Input: part model. Units: mm. Frame: model coordinates. Face numbers are marked on the shaded views. A direction names the side the tool comes from. Coordinates: 2 decimals unless noted, no trailing zeros. Order: outer loops, then holes, each group sorted by start corner. A loop starts at its lowest first (then second) coordinate and runs counter-clockwise, first axis right, second up. Notation, with made-up numbers: M -24.5,-1 L -4.5,-1 A7 cw -4.5,6 Z; hole C -3.5,28 d5. An arc over 180 degrees is marked long. Answer in a Markdown table with one row per item.
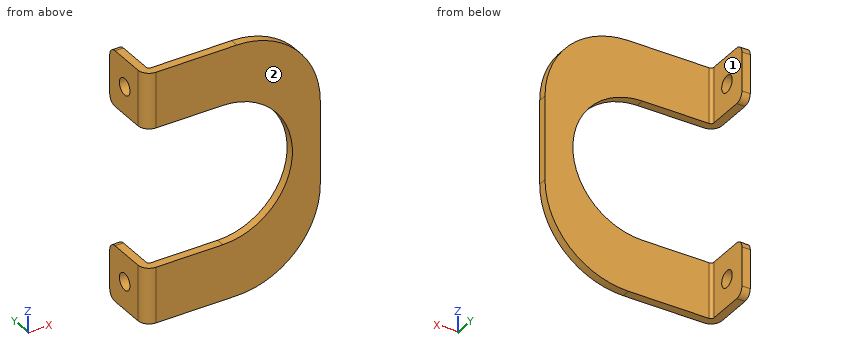
from build123d import *

# Parameters (mm, degrees)
BOSS_EXTRUDE1_DEPTH            = 3
EDGE_FLANGE1_STRIP_W           = 14
EDGE_FLANGE1_STRIP_H           = 3
EDGE_FLANGE1_STRIP_CUT_DEPTH   = 20
EDGE_FLANGE1_STRIP_2_W         = 14
EDGE_FLANGE1_STRIP_2_H         = 3
EDGE_FLANGE1_STRIP_CUT_2_DEPTH = 20
EDGE_FLANGE1_DEPTH             = 20
EDGE_FLANGE1_BEND_DEPTH        = 20
FILLET1_R                      = 3
CUT_EXTRUDE1_REACH             = 79.621
SKETCH12_R                     = 3


# Sheet-metal steps are written as plain solids
with BuildPart() as part:
    # Sketch1 → Boss-Extrude1 (new body)
    with BuildSketch(Plane(origin=(0, 0, 0), x_dir=(1, 0, 0), z_dir=(0, 1, 0))):
        with BuildLine():
            Line((0, 25), (-25, 25))
            Line((-25, 25), (-25, 45))
            Line((-25, 45), (5, 45))
            ThreePointArc((5, 45), (26.213203436, 36.213203436), (35, 15))
            Line((35, 15), (35, -15))
            ThreePointArc((35, -15), (26.213203436, -36.213203436), (5, -45))
            Line((5, -45), (-25, -45))
            Line((-25, -45), (-25, -25))
            Line((-25, -25), (0, -25))
            ThreePointArc((0, -25), (25, 0), (0, 25))
        make_face()
    extrude(amount=BOSS_EXTRUDE1_DEPTH)

    # Edge-Flange1 strip (across the edge) → Edge-Flange1 strip cut (cut)
    with BuildSketch(Plane(origin=(-25, 3, 25), x_dir=(1, 0, 0), z_dir=(0, 0, 1))):
        with Locations((-6, -1.5)):
            Rectangle(EDGE_FLANGE1_STRIP_W, EDGE_FLANGE1_STRIP_H)
    extrude(amount=EDGE_FLANGE1_STRIP_CUT_DEPTH, mode=Mode.SUBTRACT)

    # Edge-Flange1 strip 2 (across the edge) → Edge-Flange1 strip cut 2 (cut)
    with BuildSketch(Plane(origin=(-25, 3, -45), x_dir=(1, 0, 0), z_dir=(0, 0, 1))):
        with Locations((-6, -1.5)):
            Rectangle(EDGE_FLANGE1_STRIP_2_W, EDGE_FLANGE1_STRIP_2_H)
    extrude(amount=EDGE_FLANGE1_STRIP_CUT_2_DEPTH, mode=Mode.SUBTRACT)

    # Edge-Flange1 section (across the edge) → Edge-Flange1 (add)
    with BuildSketch(Plane(origin=(-25, 3, 25), x_dir=(1, 0, 0), z_dir=(0, 0, 1))):
        with BuildLine():
            Line((-3, 1), (-3, 17))
            Line((-3, 17), (0, 17))
            Line((0, 17), (0, 1))
            ThreePointArc((0, 1), (0.292893219, 0.292893219), (1, 0))
            Line((1, 0), (1, -3))
            ThreePointArc((1, -3), (-1.828427125, -1.828427125), (-3, 1))
        make_face()
    extrude(amount=EDGE_FLANGE1_DEPTH)

    # Edge-Flange1 section 2 (across the edge) → Edge-Flange1 bend (add)
    with BuildSketch(Plane(origin=(-25, 3, -45), x_dir=(1, 0, 0), z_dir=(0, 0, 1))):
        with BuildLine():
            Line((-3, 1), (-3, 17))
            Line((-3, 17), (0, 17))
            Line((0, 17), (0, 1))
            ThreePointArc((0, 1), (0.292893219, 0.292893219), (1, 0))
            Line((1, 0), (1, -3))
            ThreePointArc((1, -3), (-1.828427125, -1.828427125), (-3, 1))
        make_face()
    extrude(amount=EDGE_FLANGE1_BEND_DEPTH)

    # Fillet1
    fillet1_edges = [part.edges().sort_by_distance(p)[0] for p in [
        (-26.5, 20, 25),
        (-26.5, 20, 45),
        (-26.5, 20, -45),
        (-26.5, 20, -25),
    ]]
    fillet(fillet1_edges, radius=FILLET1_R)

    # Sketch12 → Cut-Extrude1 (cut, up to next)
    with BuildSketch(Plane(origin=(-25, 0, 0), x_dir=(0, 0, -1), z_dir=(1, 0, 0)), mode=Mode.PRIVATE) as cut_extrude1_sk1:
        with Locations(Location((35, 11.5, 0), (0, 0, 90))):
            Circle(SKETCH12_R)
    cut_extrude1_tool1 = extrude(cut_extrude1_sk1.sketch, amount=-CUT_EXTRUDE1_REACH, mode=Mode.PRIVATE) & part.part
    # Sketch12 → Cut-Extrude1 (cut, up to next)
    with BuildSketch(Plane(origin=(-25, 0, 0), x_dir=(0, 0, -1), z_dir=(1, 0, 0)), mode=Mode.PRIVATE) as cut_extrude1_sk2:
        with Locations(Location((-35, 11.5, 0), (0, 0, 90))):
            Circle(SKETCH12_R)
    cut_extrude1_tool2 = extrude(cut_extrude1_sk2.sketch, amount=-CUT_EXTRUDE1_REACH, mode=Mode.PRIVATE) & part.part
    add(cut_extrude1_tool1.solids().sort_by_distance((-25, 11.5, -35))[0], mode=Mode.SUBTRACT)
    add(cut_extrude1_tool2.solids().sort_by_distance((-25, 11.5, 35))[0], mode=Mode.SUBTRACT)


solid = part.part
1) Cut plane A-A, the plane y = 11.5. Output: boundary loops of the cut face in (x, z).
Resolved:
| item | result |
|---|---|
| outline | M -28,-45 L -25,-45 L -25,-38 L -28,-38 Z; M -28,-32 L -25,-32 L -25,-25 L -28,-25 Z; M -28,25 L -25,25 L -25,32 L -28,32 Z; M -28,38 L -25,38 L -25,45 L -28,45 Z |
2) Reachability of the marked faces 1 and 2 from +Z, -Z, +X, -X, +Y, -Y: full face, straight path, thin tool, end or side. Return the list, or none.
Resolved:
| item | result |
|---|---|
| face 1 | +Z, -Z, +X, +Y |
| face 2 | +Z, -Z, +X, -X, -Y |
3) Material intervals for probe 1 along Z at (x, y) = (-27.3, 11.5); probe 2 along Z at (x, y) = (-0.5, 1.75); probe 3 along Y at (x, z) = (7, 30), sorted ascending.
Resolved:
| item | result |
|---|---|
| probe 1 | z = -45 to -38, -32 to -25, 25 to 32, 38 to 45 |
| probe 2 | z = -45 to -25, 25 to 45 |
| probe 3 | y = 0 to 3 |
4) Cut plane B-B, the plane x = -2. Output: boundary loops of the cut face in (y, z).
Resolved:
| item | result |
|---|---|
| outline | M 0,-45 L 3,-45 L 3,-25 L 0,-25 Z; M 0,25 L 3,25 L 3,45 L 0,45 Z |
5) Cut plane D-D, the plane z = 35. Output: boundary loops of the cut face in (x, y).
Resolved:
| item | result |
|---|---|
| outline | M -28,4 A4 ccw -24,0 L 27.36,0 L 27.36,3 L -24,3 A1 cw -25,4 L -25,8.5 L -28,8.5 Z; M -28,14.5 L -25,14.5 L -25,20 L -28,20 Z |
6) Cut plane C-C, the plane y = 5.5. Output: boundary loops of the cut face in (x, z), and give its area (3 significant figures).
Resolved:
| item | result |
|---|---|
| outline | M -28,-45 L -25,-45 L -25,-25 L -28,-25 Z; M -28,25 L -25,25 L -25,45 L -28,45 Z |
| area | 120 mm2 |
7) Contact query for flat-ended pins moving along their axis: pin 1 (7 mm diameter, centred on y = 11.5, z = 35, fed in from +X); pin 2 (12 mm diameter, centred on y = 2.5, z = 2, fed in from -X); pin 3 (4 mm diameter, centred on y = 4, z = -23, fed in from +X). Output: stop coordinate, or through.
Resolved:
| item | result |
|---|---|
| pin 1 | stops at x = -25 |
| pin 2 | stops at x = 23.69 |
| pin 3 | stops at x = 34.34 |
